Here's how the part is built. I have some questions about the finished solid (model axes, mm). Give positions to 0.01 mm unless a question says otherwise; leave off trailing zeros. Write each loop counter-clockwise with the first axis right and the second up, starting at its lowest first coordinate (ties: lowest second). Pieces come first, ordered by that corner, then holes. Notation, with made-up numbers: (82.25, 45.25) -> (96.25, 45.25) arc R35 ccw to (96.25, 81.25) -> close; hole circle Ø6 at (1, -7.5). An arc over 180 degrees is marked (long way). Answer as CSV lines item,"result". Start each with the question number.
from build123d import *

# Parameters (mm, degrees)
SKETCH1_W           = 127
SKETCH1_H           = 177.8
SKETCH1_R           = 2.3749
SKETCH1_R_2         = 6.35
BOSS_EXTRUDE1_DEPTH = 10
SKETCH8_R           = 1.625
BREADBOARD_DEPTH    = 10
SKETCH9_R           = 1.75
FPGA_DEPTH          = 10
SKETCH10_R          = 1.5875
F_8PUSH_BTN_DEPTH   = 10


with BuildPart() as part:
    # Sketch1 → Boss-Extrude1 (new body)
    with BuildSketch(Plane(origin=(0, 0, 0), x_dir=(1, 0, 0), z_dir=(0, 1, 0))):
        Rectangle(SKETCH1_W, SKETCH1_H)
        with Locations(Location((-53.34, 82.55, 0), (0, 0, 270))):  # turned: the seam where the file's is
            Circle(SKETCH1_R, mode=Mode.SUBTRACT)
        with Locations(Location((53.34, 82.55, 0), (0, 0, 270))):  # turned: the seam where the file's is
            Circle(SKETCH1_R, mode=Mode.SUBTRACT)
        with Locations(Location((53.34, -82.55, 0), (0, 0, 270))):  # turned: the seam where the file's is
            Circle(SKETCH1_R, mode=Mode.SUBTRACT)
        with Locations(Location((-53.34, -82.55, 0), (0, 0, 270))):  # turned: the seam where the file's is
            Circle(SKETCH1_R, mode=Mode.SUBTRACT)
        with Locations(Location((-53.34, -38.1, 0), (0, 0, 270))):  # turned: the seam where the file's is
            Circle(SKETCH1_R_2, mode=Mode.SUBTRACT)
    extrude(amount=BOSS_EXTRUDE1_DEPTH)

    # Sketch8 → Breadboard (cut)
    with BuildSketch(Plane(origin=(0, 10, 0), x_dir=(1, 0, 0), z_dir=(0, 1, 0))):
        with Locations(Location((37, -74.5497835, 0), (0, 0, 270))):  # turned: the seam where the file's is
            Circle(SKETCH8_R)
        with Locations(Location((-37, -74.5497835, 0), (0, 0, 270))):  # turned: the seam where the file's is
            Circle(SKETCH8_R)
        with Locations(Location((-37, -41.0497835, 0), (0, 0, 270))):  # turned: the seam where the file's is
            Circle(SKETCH8_R)
        with Locations(Location((37, -41.0497835, 0), (0, 0, 270))):  # turned: the seam where the file's is
            Circle(SKETCH8_R)
    extrude(amount=-BREADBOARD_DEPTH, mode=Mode.SUBTRACT)

    # Sketch9 → FPGA (cut)
    with BuildSketch(Plane(origin=(0, 10, 0), x_dir=(1, 0, 0), z_dir=(0, 1, 0))):
        with Locations(Location((-34, 70.603714811, 0), (0, 0, 270))):  # turned: the seam where the file's is
            Circle(SKETCH9_R)
        with Locations(Location((34, 70.603714811, 0), (0, 0, 270))):  # turned: the seam where the file's is
            Circle(SKETCH9_R)
        with Locations(Location((34, 2.603714811, 0), (0, 0, 270))):  # turned: the seam where the file's is
            Circle(SKETCH9_R)
        with Locations(Location((-34, 2.603714811, 0), (0, 0, 270))):  # turned: the seam where the file's is
            Circle(SKETCH9_R)
    extrude(amount=-FPGA_DEPTH, mode=Mode.SUBTRACT)

    # Sketch10 → 8Push_btn (cut)
    with BuildSketch(Plane(origin=(0, 10, 0), x_dir=(1, 0, 0), z_dir=(0, 1, 0))):
        with Locations(Location((-25.908, -9.593705545, 0), (0, 0, 270))):  # turned: the seam where the file's is
            Circle(SKETCH10_R)
        with Locations(Location((-25.908, -26.357705545, 0), (0, 0, 270))):  # turned: the seam where the file's is
            Circle(SKETCH10_R)
        with Locations(Location((25.908, -26.357705545, 0), (0, 0, 270))):  # turned: the seam where the file's is
            Circle(SKETCH10_R)
        with Locations(Location((25.908, -9.593705545, 0), (0, 0, 270))):  # turned: the seam where the file's is
            Circle(SKETCH10_R)
    extrude(amount=-F_8PUSH_BTN_DEPTH, mode=Mode.SUBTRACT)


solid = part.part
Item 1: If we section it at B-B (x = -53.34): Please give me the cut outline in (y, z).
Item 2: If I drill on line 1 (X direction, y = 7.25, z = -82.55); line 2 (X direction, y = 3.25, z = 8.5); line 3 (X direction, y = 7, z = 38), over which ranges is the centre line in solid material (lowest first)? Write a range as [from, to].
Item 3: If we section it at A-A (z = -82.55): Please give me the cut outline in (x, y).
Item 4: I'm going to push flat-ended pins straight in: pin 1 (3 mm diameter, centred on x = 37, z = 74.55, fed in from +Y); pin 2 (7.5 mm diameter, centred on x = 53.34, z = -82.55, fed in from -Y). Where does each tip first touch, or does it pass through?
Item 5: We'd pull the mould along X, two halves only. Please class faces 1 (the face through (34.08, 5.07, -4.35)), 2 (the face through (-63.5, 5, 1)), 3 (the face through (-1, 0, -1)): released by +X, released by -X, zero draft, split by the parting line, or undercut.
Final values:
1,outline,"(0, -88.9) -> (10, -88.9) -> (10, -84.92) -> (0, -84.92) -> close; (0, -80.18) -> (10, -80.18) -> (10, 31.75) -> (0, 31.75) -> close; (0, 44.45) -> (10, 44.45) -> (10, 80.18) -> (0, 80.18) -> close; (0, 84.92) -> (10, 84.92) -> (10, 88.9) -> (0, 88.9) -> close"
2,line 1,"[-63.5, -55.71], [-50.97, 50.97], [55.71, 63.5]"
2,line 2,"[-63.5, -27.06], [-24.76, 24.76], [27.06, 63.5]"
2,line 3,"[-63.5, -59.69], [-46.99, 63.5]"
3,outline,"(-63.5, 0) -> (-55.71, 0) -> (-55.71, 10) -> (-63.5, 10) -> close; (-50.97, 0) -> (50.97, 0) -> (50.97, 10) -> (-50.97, 10) -> close; (55.71, 0) -> (63.5, 0) -> (63.5, 10) -> (55.71, 10) -> close"
4,pin 1,"through"
4,pin 2,"y = 0"
5,face 1,"undercut"
5,face 2,"released by -X"
5,face 3,"zero draft"
